The listing builds one solid part. Answer for the finished solid, in the listing's coordinates (mm). Give positions to 0.01 mm unless a question says otherwise; leave off trailing zeros. Loops run counter-clockwise (first coordinate to the right, second up) from the corner with the lowest first, then second, coordinate; pieces in that order, holes last. Notation, with made-up numbers: (82, 65.25) - (116, 65.25) arc R18 ccw to (116, 78.25) - close; hole circle Ø2 at (19, -2). An arc over 180 degrees is marked (long way). One line per item, written item: value. Start each with the question number.
from build123d import *

# Parameters (mm, degrees)
SKETCH1_R           = 1.5
BOSS_EXTRUDE1_DEPTH = 4


with BuildPart() as part:
    # Sketch1 → Boss-Extrude1 (new body)
    with BuildSketch(Plane.XY):
        with BuildLine():
            ThreePointArc((3.986498359, 25.359172843), (-2.801068394, 26.303288059), (-5.24004212, 19.899084507))
            ThreePointArc((-5.24004212, 19.899084507), (-3.822090045, 10.785), (-5.24004212, 1.670915493))
            ThreePointArc((-5.24004212, 1.670915493), (-2.801068394, -4.733288059), (3.986498359, -3.789172843))
            ThreePointArc((3.986498359, -3.789172843), (15.581947878, 3.773729824), (29.338611035, 5.324911664))
            ThreePointArc((29.338611035, 5.324911664), (35.5, 10.785), (29.338611035, 16.245088336))
            ThreePointArc((29.338611035, 16.245088336), (15.581947878, 17.796270176), (3.986498359, 25.359172843))
        make_face()
        with Locations((0, 21.57)):
            Circle(SKETCH1_R, mode=Mode.SUBTRACT)
        with Locations((30, 10.785)):
            Circle(SKETCH1_R, mode=Mode.SUBTRACT)
        Circle(SKETCH1_R, mode=Mode.SUBTRACT)
    extrude(amount=BOSS_EXTRUDE1_DEPTH)


solid = part.part
1. A cutting plane is placed at B-B (x = 0). Determine the outline of the cut face in (y, z).
2. A cutting plane is placed at C-C (y = 0). Determine the outline of the cut face in (x, z), plus the area to 3 significant figures.
3. Find the intervals of material crossed by L1, parallel to Y at x = 0, z = 3.15; L2, parallel to Y at x = 30, z = 2.1 (3 decimals); L3, parallel to X at y = 1, z = 1.25, in increasing order. Write a range as [from, to].
4. Flat-ended cylindrical pins translate along their axes: pin 1 (1.5 mm diameter, centred on y = 1, z = 1, fed in from +X); pin 2 (8 mm diameter, centred on x = 13, y = 8, fed in from -Z); pin 3 (2.5 mm diameter, centred on x = 30, y = 10.785, fed in from -Z). Find the tip coordinate at first contact, or state that the pin passes through.
5. A cutting plane is placed at A-A (x = 30). Determine the outline of the cut face in (y, z) (3 decimals), plus the area to 3 significant figures.
6. Determine the mould class of faces 1 (the cylindrical face through (15.398, 3.707, 1.972)), 2 (the cylindrical face through (-3.822, 10.915, 1.972)), 3 (the flat face through (10, 11, 0)) for opening direction X: released by +X, released by -X, zero draft, split by the parting line, or undercut.
7. A cutting plane is placed at D-D (z = 2.1). Determine the outline of the cut face in (x, y) (1 decimal).
Results below:
1. outline: (-5.5, 0) - (-1.5, 0) - (-1.5, 4) - (-5.5, 4) - close; (1.5, 0) - (20.07, 0) - (20.07, 4) - (1.5, 4) - close; (23.07, 0) - (27.07, 0) - (27.07, 4) - (23.07, 4) - close
2. outline: (-5.5, 0) - (-1.5, 0) - (-1.5, 4) - (-5.5, 4) - close; (1.5, 0) - (8.36, 0) - (8.36, 4) - (1.5, 4) - close
2. area: 43.4 mm^2
3. L1: y = [-5.5, -1.5], [1.5, 20.07], [23.07, 27.07]
3. L2: y = [5.285, 9.285], [12.285, 16.285]
3. L3: x = [-5.41, -1.12], [1.12, 9.86]
4. pin 1: stops at x = 11.13
4. pin 2: stops at z = 0
4. pin 3: passes through
5. outline: (5.285, 0) - (9.285, 0) - (9.285, 4) - (5.285, 4) - close; (12.285, 0) - (16.285, 0) - (16.285, 4) - (12.285, 4) - close
5. area: 32.0 mm^2
6. face 1: undercut
6. face 2: released by -X
6. face 3: zero draft
7. outline: (-5.2, 1.7) arc R5.5 ccw to (4, -3.8) arc R30 cw to (29.3, 5.3) arc R5.5 ccw (long way) to (29.3, 16.2) arc R30 cw to (4, 25.4) arc R5.5 ccw to (-5.2, 19.9) arc R30 cw to start; hole circle Ø3 at (0, 0); hole circle Ø3 at (0, 21.6); hole circle Ø3 at (30, 10.8)
